Design review of the part built by this model. Coordinates are the model's own, in mm. Face numbers are marked on the shaded views. A direction names the side the tool comes from. Coordinates: 2 decimals unless noted, no trailing zeros. Write each loop counter-clockwise with the first axis right and the second up, starting at its lowest first coordinate (ties: lowest second). Pieces come first, ordered by that corner, then holes.
Q1. Take a section at A-A, the plane y = 6.5. Write out the cut boundary in (x, z).
Q2. Take a section at D-D, the plane y = 4.75. Write out the cut boundary in (x, z) (3 decimals).
Q3. The part is to be moulded in two halves that separate along Z. For the marked faces 3, 4 and 5, say which applies: released by +Z, released by -Z, zero draft, split by the parting line, or undercut.
Q4. Take a section at C-C, the plane x = -1.5. Write out the cut boundary in (y, z), plus the area to 3 significant figures.
Q5. Take a section at B-B, the plane z = -10.25. Write out the cut boundary in (x, y), plus the area to 3 significant figures.
Q6. For L1, parallel to Z at x = -6.75, y = 0.5; L2, parallel to X at y = 3.55, z = -7.95 (3 decimals); L3, parallel to X at y = 1.25, z = -7.95 (3 decimals), list the stretches that pass through material, from the lowest coordinate up.
Q7. For the marked faces 1 and 2, list the 3-axis set-ups (+Z, -Z, +X, -X, +Y, -Y) from which the entire face can be reached by the end or side of a thin tool; tool diameter is ignored.
Q8. For pin 1 Ø1 at (y, z) = (5, -6) entering from -X; pin 2 Ø1 at (x, z) = (-3, -11.5) entering from +Y; pin 3 Ø1 at (y, z) = (6, -13) entering from -X, all flat-tipped, find the tip position at first contact; note any pin that passes through.
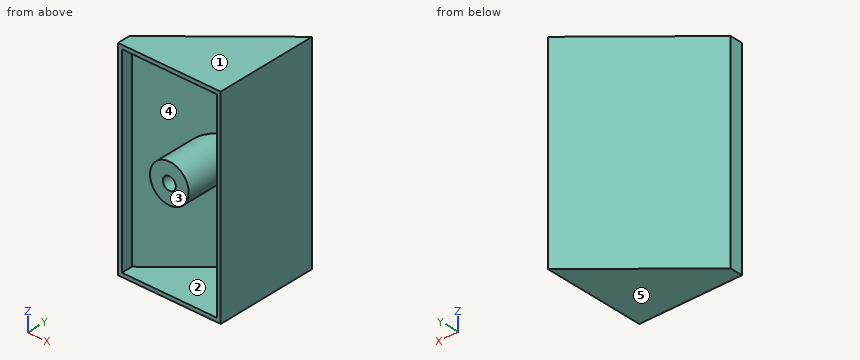
from build123d import *

# Parameters (mm, degrees)
BOSS_EXTRUDE1_DEPTH = 15.9
SHELL1_T            = -0.3
BOSS_EXTRUDE2_REACH = 21.473
SKETCH2_R           = 1.5
SKETCH2_R_2         = 0.5


with BuildPart() as part:
    # Sketch1 → Boss-Extrude1 (new body)
    with BuildSketch(Plane.XY):
        Polygon((0, 0), (0, 7.95), (-7.95, 1), (-7.95, 0), align=None)
    extrude(amount=-BOSS_EXTRUDE1_DEPTH)

    # Shell1
    shell1_openings = [part.faces().sort_by_distance(p)[0] for p in [
        (-3.975, 0, -7.95),
    ]]
    offset(amount=SHELL1_T, openings=shell1_openings, kind=Kind.INTERSECTION)

    # Boss-Extrude2: up to this plane
    boss_extrude2_end = Plane(origin=(-7.752549204, 0.774139018, -15.9), z_dir=(-0.6581693191022402, 0.7528699405557999, 0))
    # Sketch2 → Boss-Extrude2 (add, up to the surface)
    with BuildSketch(Plane(origin=(0, 0, 0), x_dir=(1, 0, 0), z_dir=(0, 1, 0)), mode=Mode.PRIVATE) as boss_extrude2_sk1:
        with Locations(Location((-3.975, 7.95, 0), (0, 0, 180))):
            Circle(SKETCH2_R)
        with Locations(Location((-3.975, 7.95, 0), (0, 0, 180))):
            Circle(SKETCH2_R_2, mode=Mode.SUBTRACT)
    boss_extrude2_tool1 = split(extrude(boss_extrude2_sk1.sketch, amount=BOSS_EXTRUDE2_REACH, mode=Mode.PRIVATE), bisect_by=boss_extrude2_end, keep=Keep.BOTH, mode=Mode.PRIVATE)
    add(boss_extrude2_tool1.solids().sort_by_distance((-2.517426, 0, -7.95))[0])


solid = part.part
Responses:
1. outline: (-1.66, -15.9) - (0, -15.9) - (0, 0) - (-1.66, 0) - close; hole (-1.2, -15.6) - (-0.3, -15.6) - (-0.3, -0.3) - (-1.2, -0.3) - close
2. outline: (-3.66, -15.9) - (0, -15.9) - (0, 0) - (-3.66, 0) - close; hole (-3.205, -15.6) - (-0.3, -15.6) - (-0.3, -0.3) - (-3.205, -0.3) - (-3.205, -6.663) arc R1.5 cw to (-3.205, -9.237) - close
3. face 3: zero draft
3. face 4: undercut
3. face 5: released by -Z
4. outline: (0, -15.9) - (6.64, -15.9) - (6.64, 0) - (0, 0) - (0, -0.3) - (6.24, -0.3) - (6.24, -15.6) - (0, -15.6) - close
4. area: 10.1 mm2
5. outline: (-7.95, 0) - (-7.65, 0) - (-7.65, 0.86) - (-0.3, 7.29) - (-0.3, 0) - (0, 0) - (0, 7.95) - (-7.95, 1) - close
5. area: 5.61 mm2
6. L1: z = -15.9 to -15.6, -0.3 to 0
6. L2: x = -5.033 to -4.475, -3.475 to -2.475, -0.3 to 0
6. L3: x = -7.664 to -7.208, -5.475 to -4.475, -3.475 to -2.475, -0.3 to 0
7. face 1: +Z, +X, -X, +Y, -Y
7. face 2: -Y
8. pin 1: stops at x = -3.95
8. pin 2: stops at y = 5.76
8. pin 3: stops at x = -2.8
